from build123d import *

# Parameters (mm, degrees)
BOSS_EXTRUDE1_DEPTH = 67
SKETCH2_W           = 103
SKETCH2_H           = 142
BOSS_EXTRUDE2_DEPTH = 9
SKETCH3_W           = 90
SKETCH3_H           = 2
BOSS_EXTRUDE3_DEPTH = 4
SKETCH4_W           = 93
SKETCH4_H           = 24
BOSS_EXTRUDE4_DEPTH = 26
BOSS_EXTRUDE5_DEPTH = 93
BOSS_EXTRUDE6_REACH = 161.108
BOSS_EXTRUDE7_DEPTH = 93
SHELL5_START        = -44.5
SHELL5_DEPTH        = 89
SHELL5_START_2      = -49.5
SHELL5_2_DEPTH      = 99
SHELL5_3_OUTLINE_W  = 67
SHELL5_3_OUTLINE_H  = 4
SHELL5_3_DEPTH      = 21.298437881
SHELL5_START_3      = 23.201562119
SHELL5_4_OUTLINE_W  = 67
SHELL5_4_OUTLINE_H  = 4
SHELL5_4_DEPTH      = 21.298437881
SHELL5_START_4      = 2
SHELL5_5_DEPTH      = 67
CUT_EXTRUDE1_REACH  = 193.448
SKETCH11_W          = 99
SKETCH11_H          = 41
FILLET2_R           = 1
SKETCH12_W          = 2
SKETCH12_H          = 67
BOSS_EXTRUDE8_DEPTH = 2
SKETCH13_W          = 76
SKETCH13_H          = 4
BOSS_EXTRUDE9_DEPTH = 4


with BuildPart() as part:
    # Sketch1 → Boss-Extrude1 (new body)
    with BuildSketch(Plane(origin=(0, 0, 0), x_dir=(1, 0, 0), z_dir=(0, 1, 0))):
        Polygon((-17.5, 64.5), (17.5, 64.5), (22.5, 68.5), (46.5, 68.5), (46.5, -68.5), (-46.5, -68.5), (-46.5, 68.5), (-22.5, 68.5), align=None)
    extrude(amount=BOSS_EXTRUDE1_DEPTH)

    # Sketch2 → Boss-Extrude2 (add)
    with BuildSketch(Plane(origin=(0, 67, 0), x_dir=(1, 0, 0), z_dir=(0, 1, 0))):
        with Locations((0, 2.5)):
            Rectangle(SKETCH2_W, SKETCH2_H)
    extrude(amount=BOSS_EXTRUDE2_DEPTH)

    # Sketch3 → Boss-Extrude3 (add)
    with BuildSketch(Plane.XZ.offset(-67)):
        with Locations((0, -72.5)):
            Rectangle(SKETCH3_W, SKETCH3_H)
    extrude(amount=BOSS_EXTRUDE3_DEPTH)

    # Sketch4 → Boss-Extrude4 (add)
    with BuildSketch(Plane.XY.offset(68.5)):
        with Locations((0, 21)):
            Rectangle(SKETCH4_W, SKETCH4_H)
    extrude(amount=BOSS_EXTRUDE4_DEPTH)

    # Sketch5 → Boss-Extrude5 (add)
    with BuildSketch(Plane.ZY.offset(46.5)):
        Polygon((68.5, 67), (94.5, 33), (68.5, 33), align=None)
    extrude(amount=-BOSS_EXTRUDE5_DEPTH)

    # Boss-Extrude6: up to this face of the body (flat: up to its plane)
    boss_extrude6_end = Plane(part.part.faces().sort_by_distance((51.5, 71.5, -2.5))[0])
    # Sketch7 → Boss-Extrude6 (add, up to the picked face)
    with BuildSketch(Plane.ZY.offset(51.5), mode=Mode.PRIVATE) as boss_extrude6_sk1:
        Polygon((68.5, 67), (84.547855551, 33), (94.5, 33), (74.204182686, 76), (68.5, 76), align=None)
    boss_extrude6_tool1 = split(extrude(boss_extrude6_sk1.sketch, amount=-BOSS_EXTRUDE6_REACH, mode=Mode.PRIVATE), bisect_by=boss_extrude6_end, keep=Keep.BOTH, mode=Mode.PRIVATE)
    add(boss_extrude6_tool1.solids().sort_by(Axis((-51.5, 53.63498, 79.950766), (1, 0, 0)))[0])

    # Sketch8 → Boss-Extrude7 (add)
    with BuildSketch(Plane.ZY.offset(46.5)):
        with BuildLine():
            Line((76.5, 9), (68.5, 9))
            Line((68.5, 9), (68.5, 1))
            ThreePointArc((68.5, 1), (74.156854249, 3.343145751), (76.5, 9))
        make_face()
    extrude(amount=-BOSS_EXTRUDE7_DEPTH)

    # Shell5: read off the stored shape, not the designer's step
    # Shell5 outline → Shell5 (cut)
    with BuildSketch(Plane.YZ.offset(SHELL5_START)):
        with BuildLine():
            Line((69, -71.5), (76, -71.5))
            Line((76, -71.5), (76, 71.992595031))
            Line((76, 71.992595031), (32.551717034, 92.5))
            Line((32.551717034, 92.5), (11, 92.5))
            Line((11, 92.5), (11, 74.156854249))
            ThreePointArc((11, 74.156854249), (4.757359313, 72.742640687), (3.343145751, 66.5))
            Line((3.343145751, 66.5), (2, 66.5))
            Line((2, 66.5), (2, -62.5))
            Line((2, -62.5), (69, -62.5))
            Line((69, -62.5), (69, -71.5))
        make_face()
    extrude(amount=SHELL5_DEPTH, mode=Mode.SUBTRACT)

    # Shell5 2 outline → Shell5 2 (cut)
    with BuildSketch(Plane.YZ.offset(SHELL5_START_2)):
        Polygon((69, -71.5), (76, -71.5), (76, 71.992595031), (35, 91.344420842), (35, 85.815451703), (69, 69.767596152), align=None)
    extrude(amount=SHELL5_2_DEPTH, mode=Mode.SUBTRACT)

    # Shell5 3 outline → Shell5 3 (cut)
    with BuildSketch(Plane.YZ.offset(SHELL5_START)):
        with Locations((35.5, -64.5)):
            Rectangle(SHELL5_3_OUTLINE_W, SHELL5_3_OUTLINE_H)
    extrude(amount=SHELL5_3_DEPTH, mode=Mode.SUBTRACT)

    # Shell5 4 outline → Shell5 4 (cut)
    with BuildSketch(Plane.YZ.offset(SHELL5_START_3)):
        with Locations((35.5, -64.5)):
            Rectangle(SHELL5_4_OUTLINE_W, SHELL5_4_OUTLINE_H)
    extrude(amount=SHELL5_4_DEPTH, mode=Mode.SUBTRACT)

    # Shell5 5 outline → Shell5 5 (cut)
    with BuildSketch(Plane(origin=(0, 0, 0), x_dir=(1, 0, 0), z_dir=(0, 1, 0)).offset(SHELL5_START_4)):
        Polygon((-23.201562119, 62.5), (-18.201562119, 62.5), (-23.201562119, 66.5), align=None)
        Polygon((23.201562119, 66.5), (18.201562119, 62.5), (23.201562119, 62.5), align=None)
    extrude(amount=SHELL5_5_DEPTH, mode=Mode.SUBTRACT)

    # Cut-Extrude1: up to this face of the body (flat: up to its plane)
    cut_extrude1_end = Plane(part.part.faces().sort_by_distance((-47, 52, 77.791523927))[0])
    # Sketch11 → Cut-Extrude1 (cut, up to the picked face)
    with BuildSketch(Plane.XY.offset(94.5), mode=Mode.PRIVATE) as cut_extrude1_sk1:
        with Locations((0, 55.5)):
            Rectangle(SKETCH11_W, SKETCH11_H)
    cut_extrude1_tool1 = split(extrude(cut_extrude1_sk1.sketch, amount=-CUT_EXTRUDE1_REACH, mode=Mode.PRIVATE), bisect_by=cut_extrude1_end, keep=Keep.BOTH, mode=Mode.PRIVATE)
    add(cut_extrude1_tool1.solids().sort_by(Axis((0, 55.5, 94.5), (0, 0, -1)))[0], mode=Mode.SUBTRACT)

    # Fillet2
    fillet2_edges = [part.edges().sort_by_distance(p)[0] for p in [
        (0, 35, 93.556008497),
    ]]
    fillet(fillet2_edges, radius=FILLET2_R)

    # Sketch12 → Boss-Extrude8 (add)
    with BuildSketch(Plane.ZY.offset(46.5)):
        with Locations((-57.5, 33.5)):
            Rectangle(SKETCH12_W, SKETCH12_H)
        with Locations((-53.5, 33.5)):
            Rectangle(SKETCH12_W, SKETCH12_H)
        with Locations((-49.5, 33.5)):
            Rectangle(SKETCH12_W, SKETCH12_H)
        with Locations((59.5, 33.5)):
            Rectangle(SKETCH12_W, SKETCH12_H)
        with Locations((63.5, 33.5)):
            Rectangle(SKETCH12_W, SKETCH12_H)
        with Locations((67.5, 33.5)):
            Rectangle(SKETCH12_W, SKETCH12_H)
    boss_extrude8 = extrude(amount=BOSS_EXTRUDE8_DEPTH)

    # Mirror1: Boss-Extrude8 across plane
    add(boss_extrude8.mirror(Plane(origin=(0, 0, 0), x_dir=(0, 0, 1), z_dir=(1, 0, 0))))

    # Sketch13 → Boss-Extrude9 (add)
    with BuildSketch(Plane.XY.offset(94.5)):
        Polygon((-42, 32), (-42, 9), (-38, 9), (-38, 13), (-38, 32), align=None)
        with Locations((0, 11)):
            Rectangle(SKETCH13_W, SKETCH13_H)
        Polygon((38, 13), (38, 9), (42, 9), (42, 32), (38, 32), align=None)
    extrude(amount=BOSS_EXTRUDE9_DEPTH)


solid = part.part
Work out the finished part from the listing and answer in its coordinate system (mm). A direction names the side the tool comes from. Give positions to 0.01 mm unless a question says otherwise; leave off trailing zeros. Order: outer loops, then holes, each group sorted by start corner. A loop starts at its lowest first (then second) coordinate and runs counter-clockwise, first axis right, second up. Notation, with made-up numbers: (61, -38) -> (98, -38) arc R19 ccw to (98, -28) -> close; hole circle Ø3 at (-15, -34.75). An arc over 180 degrees is marked (long way). One line per item, written item: value.
Item 1: Straight lines are drawn through the part: probe 1 along X at (y, z) = (45, -57); probe 2 along Z at (x, y) = (6.5, 24); probe 3 along X at (y, z) = (7.5, -52). For each, find the intervals that lie inside material, in ascending order.
Answer sheet:
probe 1: -48.5 to -44.5, 44.5 to 48.5
probe 2: -64.5 to -62.5, 92.5 to 94.5
probe 3: -46.5 to -44.5, 44.5 to 46.5
Item 2: Flat-ended cylindrical pins translate along their axes: P1, Ø2, axis at y = 22, z = 96, coming from the -X side; P2, Ø2, axis at y = 42, z = 63, coming from the +X side; P3, Ø5, axis at x = -28.5, z = 16, coming from the -Y side; P4, Ø0.6, axis at y = 28, z = 63.5, coming from the -X side. Find the tip coordinate at first contact, or state that the pin passes through.
Answer sheet:
P1: x = -42
P2: x = 48.5
P3: y = 0
P4: x = -48.5
Item 3: Determine the mould class of faces 1 (the flat face through (-1, 2, 1)), 2 (the cylindrical face through (-0.651, 3.281, 74.094)), 3 (the flat face through (-1, 13, 96)) for opening direction Z: released by +Z, released by -Z, zero draft, split by the parting line, or undercut.
Answer sheet:
face 1: undercut
face 2: released by +Z
face 3: zero draft
Item 4: Find section A-A, the plane z = -12.5. Give the vertices of the cut face in (x, y), plus the area to 3 significant figures.
Answer sheet:
outline: (-51.5, 67) -> (-46.5, 67) -> (-46.5, 0) -> (46.5, 0) -> (46.5, 67) -> (51.5, 67) -> (51.5, 76) -> (49.5, 76) -> (49.5, 69) -> (44.5, 69) -> (44.5, 2) -> (-44.5, 2) -> (-44.5, 69) -> (-49.5, 69) -> (-49.5, 76) -> (-51.5, 76) -> close
area: 502 mm²
Item 5: Find section B-B, the plane x = -4.5. Give the vertices of the cut face in (y, z).
Answer sheet:
outline: (0, -64.5) -> (67, -64.5) -> (67, -71.5) -> (63, -71.5) -> (63, -73.5) -> (76, -73.5) -> (76, -71.5) -> (69, -71.5) -> (69, -62.5) -> (2, -62.5) -> (2, 66.5) -> (3.34, 66.5) arc R6 cw to (11, 74.16) -> (11, 92.5) -> (32.55, 92.5) -> (35, 91.34) -> (35, 92.92) arc R1 ccw to (34.43, 93.83) -> (33, 94.5) -> (13, 94.5) -> (13, 98.5) -> (9, 98.5) -> (9, 76.5) arc R8 ccw to (1, 68.5) -> (0, 68.5) -> close
Item 6: A tool of negligible diameter and unlimited length cuts with its end or side. For faces 4 (the flat face through (-46.5, 34, -64)), 5 (the flat face through (20.7, 35, -64.5)), 6 (the flat face through (-38, 22, 96)), 7 (the flat face through (-42, 21, 96)), 8 (the cylindrical face through (-0.623, 4.825, 72.809)), from which of +Z, -Z, +X, -X, +Y, -Y can it reach the whole face along a straight path? Write none if from no direction.
Answer sheet:
face 4: -Z, -X, -Y
face 5: +Y
face 6: +Z, +Y
face 7: +Z, -X, +Y, -Y
face 8: none
